from build123d import *

# Parameters (mm, degrees)
SKETCH1_W           = 25.4
SKETCH1_H           = 50.8
SKETCH1_W_2         = 19.05
SKETCH1_H_2         = 44.45
BOSS_EXTRUDE1_DEPTH = 457.2
SKETCH2_R           = 14.2875
CUT_EXTRUDE1_DEPTH  = 26.4


with BuildPart() as part:
    # Sketch1 → Boss-Extrude1 (new body)
    with BuildSketch(Plane.XY):
        with Locations((12.7, 25.4)):
            Rectangle(SKETCH1_W, SKETCH1_H)
        with Locations((12.7, 25.4)):
            Rectangle(SKETCH1_W_2, SKETCH1_H_2, mode=Mode.SUBTRACT)
    extrude(amount=BOSS_EXTRUDE1_DEPTH)

    # Sketch2 → Cut-Extrude1 (cut, through all)
    with BuildSketch(Plane(origin=(25.4, 0, 0), x_dir=(0, 0, -1), z_dir=(1, 0, 0))):
        with Locations((-406.4, 25.4)):
            Circle(SKETCH2_R)
        with Locations((-203.2, 25.4)):
            Circle(SKETCH2_R)
    extrude(amount=-CUT_EXTRUDE1_DEPTH, mode=Mode.SUBTRACT)


solid = part.part
Can you work these out from the model? Positions are in its coordinate system, mm. A direction names the side the tool comes from. Coordinates: 2 decimals unless noted, no trailing zeros. Write each loop counter-clockwise with the first axis right and the second up, starting at its lowest first coordinate (ties: lowest second). Pieces come first, ordered by that corner, then holes. Notation, with made-up numbers: (5.5, 37.25) - (13.5, 37.25) arc R12 cw to (13.5, 56.25) - close; hole circle Ø8 at (75.25, 53). An arc over 180 degrees is marked (long way). Return JSON: item names as keys, results as strings. Group by question number.
Item 1: If we section it at C-C (y = 25.4): Write out the boundary of the cut face in (x, z) (1 decimal), then the cut area to 3 significant figures.
Item 2: If we section it at B-B (z = 369): Write out the boundary of the cut face in (x, y) (3 decimals).
Item 3: Which directions (+Z, -Z, +X, -X, +Y, -Y) give clear straight access to the entire face, cutting with the end or side of a thin tool? Please do faces 4 (the face through (3.175, 25, 225)), 5 (the face through (2, 24, 0)).
Item 4: If we section it at D-D (z = 203.2): Write out the boundary of the cut face in (x, y) (1 decimal), then the cut area to 3 significant figures.
Item 5: I'm going to push flat-ended pins straight in: pin 1 Ø12 at (x, y) = (14, 23) entering from -Z; pin 2 Ø5 at (x, y) = (22.5, 41.5) entering from -Z. Where does each tip first touch, or does it pass through?
Item 6: We'd pull the mould along Y, two halves only. Please class faces 1 (the face through (13, 47.625, 225)), 2 (the face through (2, 24, 457.2)), 3 (the face through (13, 50.8, 225)): pulls with the +Y half, pulls with the -Y half, needs draft (parallel to the pull), parting line crosses it, or undercut.
Item 7: If we section it at A-A (x = 14): Write out the boundary of the cut face in (y, z) (3 decimals).
Item 8: Please list where these lines run through material, in increasing order: probe 1 along Y at (x, z) = (23.6, 203.2); probe 2 along X at (y, z) = (22.5, 187.5) (3 decimals); probe 3 along Y at (x, z) = (16.5, 79) (3 decimals).
Return value:
{
 "1": {"outline": "(0, 0) - (3.2, 0) - (3.2, 188.9) - (0, 188.9) - close; (0, 217.5) - (3.2, 217.5) - (3.2, 392.1) - (0, 392.1) - close; (0, 420.7) - (3.2, 420.7) - (3.2, 457.2) - (0, 457.2) - close; (22.2, 0) - (25.4, 0) - (25.4, 188.9) - (22.2, 188.9) - close; (22.2, 217.5) - (25.4, 217.5) - (25.4, 392.1) - (22.2, 392.1) - close; (22.2, 420.7) - (25.4, 420.7) - (25.4, 457.2) - (22.2, 457.2) - close", "area": "2,540 mm^2"},
 "2": {"outline": "(0, 0) - (25.4, 0) - (25.4, 50.8) - (0, 50.8) - close; hole (3.175, 3.175) - (22.225, 3.175) - (22.225, 47.625) - (3.175, 47.625) - close"},
 "3": {"face 4": "+Z, -Z", "face 5": "-Z, +X, -X, +Y, -Y"},
 "4": {"outline": "(0, 0) - (25.4, 0) - (25.4, 11.1) - (22.2, 11.1) - (22.2, 3.2) - (3.2, 3.2) - (3.2, 11.1) - (0, 11.1) - close; (0, 39.7) - (3.2, 39.7) - (3.2, 47.6) - (22.2, 47.6) - (22.2, 39.7) - (25.4, 39.7) - (25.4, 50.8) - (0, 50.8) - close", "area": "262 mm^2"},
 "5": {"pin 1": "passes through", "pin 2": "stops at z = 0"},
 "6": {"face 1": "undercut", "face 2": "needs draft", "face 3": "pulls with the +Y half"},
 "7": {"outline": "(0, 0) - (3.175, 0) - (3.175, 457.2) - (0, 457.2) - close; (47.625, 0) - (50.8, 0) - (50.8, 457.2) - (47.625, 457.2) - close"},
 "8": {"probe 1": "y = 0 to 11.11, 39.69 to 50.8", "probe 2": "x = 0 to 3.175, 22.225 to 25.4", "probe 3": "y = 0 to 3.175, 47.625 to 50.8"}
}
